Read the model definition and answer for the solid it produces. Units are mm, in the model's axes. A direction names the side the tool comes from. Coordinates: 2 decimals unless noted, no trailing zeros. Order: outer loops, then holes, each group sorted by start corner. A loop starts at its lowest first (then second) coordinate and runs counter-clockwise, first axis right, second up. Notation, with made-up numbers: (6, -4.75) -> (24, -4.75) arc R19 cw to (24, 27.25) -> close; hole circle Ø8 at (-5, 30). An arc over 180 degrees is marked (long way). Answer as a JSON object with one key per item and string values. Group by question number.
1) Determine the mould class of faces 5 (the flat face through (-136, 89, 59)), 6 (the flat face through (-114, 44, 59)), 7 (the cylindrical face through (-1.479, 62.973, 43.859)), 8 (the cylindrical face through (-13.04, 1.48, 81.23)) for opening direction Y: released by +Y, released by -Y, zero draft, split by the parting line, or undercut.
2) Section D-D on x = -130 is taken. Determine the outline of the cut face in (y, z), and give its area (3 significant figures).
3) Section C-C on y = 55 is taken. Determine the outline of the cut face in (x, z), and give its area (3 significant figures).
4) Section B-B on x = -99 is taken. Determine the outline of the cut face in (y, z).
5) Consider L1, parallel to Z at x = -158.9, y = 66; L2, parallel to X at y = 34, z = 97; L3, parallel to Z at x = -74, y = 0.8. Determine where each line is inside the solid, lowest interval first.
6) Section A-A on z = 35 is taken. Count the separate pieces of the cut face and the enclosed holes in it, and give its area (3 significant figures).
7) A tool of negligible diameter and unlimited length cuts with its end or side. For faces 1 (the flat face through (-136, 3, 59)), 2 (the cylindrical face through (-1.479, 24.253, 12.121)), 3 (the cylindrical face through (-12.715, 1.479, 38.584)), 4 (the cylindrical face through (-159.521, 28.747, 23.121)), from which of +Z, -Z, +X, -X, +Y, -Y can it reach the whole face along a straight path? Write none if from no direction.
from build123d import *

# Parameters (mm, degrees)
SKETCH_W        = 44
SKETCH_H        = 83
PAD_DEPTH       = 120
SKETCH001_R     = 2.75
POCKET_DEPTH    = 3
SKETCH002_R     = 4.25
POCKET001_DEPTH = 3
SKETCH003_R     = 2.75
POCKET002_DEPTH = 3


with BuildPart() as part:
    # Sketch → Pad (new body)
    with BuildSketch(Plane.XY):
        Polygon((0, 0), (-161, 0), (-161, 89), (-111, 89), (-111, 3), (-3, 3), (-3, 86), (-15, 86), (-15, 89), (0, 89), align=None)
        with Locations((-136, 44.5)):
            Rectangle(SKETCH_W, SKETCH_H, mode=Mode.SUBTRACT)
    extrude(amount=PAD_DEPTH)

    # Sketch001 (on Face2 of Pad) → Pocket (cut)
    with BuildSketch(Plane.YZ):
        with Locations((27, 42)):
            Circle(SKETCH001_R)
        with Locations((65, 42)):
            Circle(SKETCH001_R)
        with Locations((27, 12)):
            Circle(SKETCH001_R)
        with Locations((65, 12)):
            Circle(SKETCH001_R)
    extrude(amount=-POCKET_DEPTH, mode=Mode.SUBTRACT)

    # Sketch002 (on Face6 of Pocket) → Pocket001 (cut)
    with BuildSketch(Plane.XZ):
        with Locations((-40, 85)):
            Circle(SKETCH002_R)
        with Locations((-15, 85)):
            Circle(SKETCH002_R)
        with Locations((-40, 35)):
            Circle(SKETCH002_R)
        with Locations((-15, 35)):
            Circle(SKETCH002_R)
        with Locations((-99, 85)):
            Circle(SKETCH002_R)
        with Locations((-74, 85)):
            Circle(SKETCH002_R)
        with Locations((-99, 35)):
            Circle(SKETCH002_R)
        with Locations((-74, 35)):
            Circle(SKETCH002_R)
    extrude(amount=-POCKET001_DEPTH, mode=Mode.SUBTRACT)

    # Sketch003 (on Face12 of Pocket001) → Pocket002 (cut)
    with BuildSketch(Plane(origin=(-161, 0, 0), x_dir=(0, -1, 0), z_dir=(-1, 0, 0))):
        with Locations((-66, 47)):
            Circle(SKETCH003_R)
        with Locations((-26, 47)):
            Circle(SKETCH003_R)
        with Locations((-66, 23)):
            Circle(SKETCH003_R)
        with Locations((-26, 23)):
            Circle(SKETCH003_R)
    extrude(amount=-POCKET002_DEPTH, mode=Mode.SUBTRACT)


solid = part.part
Worked answers:
{
 "1": {"face 5": "released by +Y", "face 6": "undercut", "face 7": "undercut", "face 8": "zero draft"},
 "2": {"outline": "(0, 0) -> (3, 0) -> (3, 120) -> (0, 120) -> close; (86, 0) -> (89, 0) -> (89, 120) -> (86, 120) -> close", "area": "720 mm²"},
 "3": {"outline": "(-161, 0) -> (-158, 0) -> (-158, 120) -> (-161, 120) -> close; (-114, 0) -> (-111, 0) -> (-111, 120) -> (-114, 120) -> close; (-3, 0) -> (0, 0) -> (0, 120) -> (-3, 120) -> close", "area": "1,080 mm²"},
 "4": {"outline": "(0, 0) -> (3, 0) -> (3, 30.75) -> (0, 30.75) -> close; (0, 39.25) -> (3, 39.25) -> (3, 80.75) -> (0, 80.75) -> close; (0, 89.25) -> (3, 89.25) -> (3, 120) -> (0, 120) -> close"},
 "5": {"L1": "z = 0 to 20.25, 25.75 to 44.25, 49.75 to 120", "L2": "x = -161 to -158, -114 to -111, -3 to 0", "L3": "z = 0 to 30.75, 39.25 to 80.75, 89.25 to 120"},
 "6": {"separate pieces": "5", "enclosed holes": "1", "area": "1,320 mm²"},
 "7": {"face 1": "+Z, -Z", "face 2": "+X", "face 3": "-Y", "face 4": "-X"}
}
